from build123d import *

# Parameters (mm, degrees)
SKETCH003_R     = 1.2
PAD001_DEPTH    = 10
POCKET002_DEPTH = 200
SKETCH011_R     = 1.2
POCKET008_DEPTH = 10
SKETCH030_W     = 5
SKETCH030_H     = 10
PAD012_DEPTH    = 2
SKETCH031_W     = 5
SKETCH031_H     = 1
POCKET018_DEPTH = 200


with BuildPart() as part:
    # Sketch003 → Pad001 (new body)
    with BuildSketch(Plane.XY):
        Polygon((-99.96, 100), (99.96, 100), (99.96, -100), (77.96, -100), (77.96, 80), (-77.96, 80), (-77.96, -100), (-99.96, -100), align=None)
        with Locations((-88.96, 80)):
            Circle(SKETCH003_R, mode=Mode.SUBTRACT)
        with Locations((88.96, 80)):
            Circle(SKETCH003_R, mode=Mode.SUBTRACT)
        with Locations((88.96, 20)):
            Circle(SKETCH003_R, mode=Mode.SUBTRACT)
        with Locations((-88.96, 20)):
            Circle(SKETCH003_R, mode=Mode.SUBTRACT)
        with Locations((-88.96, -40)):
            Circle(SKETCH003_R, mode=Mode.SUBTRACT)
        with Locations((88.96, -40)):
            Circle(SKETCH003_R, mode=Mode.SUBTRACT)
    extrude(amount=-PAD001_DEPTH)

    # Sketch004 (on Face6 of Pad001) → Pocket002 (cut)
    with BuildSketch(Plane(origin=(0, 100, 0), x_dir=(-1, 0, 0), z_dir=(0, 1, 0))):
        Polygon((-85.46, 0), (-85.46, -1), (-92.46, -1), (-92.46, 1), (92.46, 1), (92.46, -1), (85.46, -1), (85.46, 0), align=None)
    extrude(amount=-POCKET002_DEPTH, mode=Mode.SUBTRACT)

    # Sketch011 (on Face5 of Pocket002) → Pocket008 (cut)
    with BuildSketch(Plane(origin=(0, 0, -10), x_dir=(1, 0, 0), z_dir=(0, 0, -1))):
        with Locations((-79.96, -86.5)):
            Circle(SKETCH011_R)
        with Locations((-69.96, -86.5)):
            Circle(SKETCH011_R)
        with Locations((-69.96, -96.5)):
            Circle(SKETCH011_R)
        with Locations((-79.96, -96.5)):
            Circle(SKETCH011_R)
        with Locations((69.96, -86.5)):
            Circle(SKETCH011_R)
        with Locations((79.96, -86.5)):
            Circle(SKETCH011_R)
        with Locations((79.96, -96.5)):
            Circle(SKETCH011_R)
        with Locations((69.96, -96.5)):
            Circle(SKETCH011_R)
    extrude(amount=-POCKET008_DEPTH, mode=Mode.SUBTRACT)

    # Sketch030 (on Face4 of Pocket008) → Pad012 (join)
    with BuildSketch(Plane.XY):
        with Locations((97.46, 91.25)):
            Rectangle(SKETCH030_W, SKETCH030_H)
        with Locations((97.46, -91.25)):
            Rectangle(SKETCH030_W, SKETCH030_H)
        with Locations((-97.46, 91.25)):
            Rectangle(SKETCH030_W, SKETCH030_H)
        with Locations((-97.46, -91.25)):
            Rectangle(SKETCH030_W, SKETCH030_H)
    extrude(amount=PAD012_DEPTH)

    # Sketch031 (on Face2 of Pad012) → Pocket018 (cut)
    with BuildSketch(Plane.XZ.offset(100)):
        with Locations((81.71, -0.5)):
            Rectangle(SKETCH031_W, SKETCH031_H)
        with Locations((-81.71, -0.5)):
            Rectangle(SKETCH031_W, SKETCH031_H)
    extrude(amount=-POCKET018_DEPTH, mode=Mode.SUBTRACT)


with BuildPart() as part_1:
    # Body001 placement: moved
    add(part.part.moved(Location((0, 0, -34))))


solid = part_1.part
For this review, take the finished solid that the model builds, in its own axes (mm). A direction names the side the tool comes from. Coordinates: 2 decimals unless noted, no trailing zeros. Loops run counter-clockwise (first coordinate to the right, second up) from the corner with the lowest first, then second, coordinate; pieces in that order, holes last. Notation, with made-up numbers: (42.25, -24) - (49.25, -24) arc R19 ccw to (49.25, -17) - close; hole circle Ø10 at (60.5, -35.75). An arc over 180 degrees is marked (long way). Return JSON: item names as keys, results as strings.
Item 1: Take a section at A-A (z = -40). State how many separate pieces and enclosed holes the cut face has, then the cut area to 3 significant figures.
Determined:
{"separate pieces": "1", "enclosed holes": "14", "area": "11,900 mm2"}
Item 2: Take a section at C-C (x = -21.5). Give the boundary of the cut face in (y, z), then the cut area to 3 significant figures.
Determined:
{"outline": "(80, -44) - (100, -44) - (100, -34) - (80, -34) - close", "area": "200 mm2"}
Item 3: Mouldability with a two-part tool opening along Y and no side actions: class faces 1 (the flat face through (-96, 1, -34)), 2 (the flat face through (-89, 1, -35)), 3 (the flat face through (-1, 100, -39)), 4 (the flat face through (96, 1, -34)) as pulls with the +Y half, pulls with the -Y half, needs draft (parallel to the pull), parting line crosses it, or undercut.
Determined:
{"face 1": "undercut", "face 2": "needs draft", "face 3": "pulls with the +Y half", "face 4": "undercut"}
Item 4: For faces 5 (the flat face through (89, -100, -39)), 6 (the flat face through (89, 1, -35)), 7 (the flat face through (1, 80, -39)), list the 3-axis set-ups (+Z, -Z, +X, -X, +Y, -Y) from which the entire face can be reached by the end or side of a thin tool; tool diameter is ignored.
Determined:
{"face 5": "+Z, -Z, +X, -X, -Y", "face 6": "+Z, +Y, -Y", "face 7": "+Z, -Z, -Y"}
Item 5: Take a section at B-B (y = -50). Give the boundary of the cut face in (x, z).
Determined:
{"outline": "(-99.96, -44) - (-77.96, -44) - (-77.96, -34) - (-79.21, -34) - (-79.21, -35) - (-84.21, -35) - (-84.21, -34) - (-85.46, -34) - (-85.46, -35) - (-92.46, -35) - (-92.46, -34) - (-99.96, -34) - close; (77.96, -44) - (99.96, -44) - (99.96, -34) - (92.46, -34) - (92.46, -35) - (85.46, -35) - (85.46, -34) - (84.21, -34) - (84.21, -35) - (79.21, -35) - (79.21, -34) - (77.96, -34) - close"}
Item 6: For line 1 (X direction, y = 96.5, z = -40.25); line 2 (Y direction, x = -88.96, z = -39.25); line 3 (X direction, y = 25, z = -39.25), list the stretches that pass through material, from the lowest coordinate up.
Determined:
{"line 1": "x = -99.96 to -81.16, -78.76 to -71.16, -68.76 to 68.76, 71.16 to 78.76, 81.16 to 99.96", "line 2": "y = -100 to -41.2, -38.8 to 18.8, 21.2 to 78.8, 81.2 to 100", "line 3": "x = -99.96 to -77.96, 77.96 to 99.96"}
Item 7: Insertion check: pin 1 (1 mm diameter, centred on x = -98, z = -33, fed in from +Y); pin 2 (7.5 mm diameter, centred on x = 88.5, y = 2.5, fed in from +Z); pin 3 (4 mm diameter, centred on x = -88.96, y = 80, fed in from +Z). Each pin has a flat end and moves straight along its axis. Give the tip position at first contact, or say it passes through.
Determined:
{"pin 1": "stops at y = 96.25", "pin 2": "stops at z = -34", "pin 3": "stops at z = -35"}
